```python
from build123d import *

# Parameters (mm, degrees)
F1_DEPTH    = 279.4
F2_T1_DEPTH = 136.906


# Not quite as in the source:
# - a fillet or chamfer that OpenCascade refuses, or shapes differently, is made with other operations: its cross-section is extruded or revolved along the edge and cut away or added


with BuildPart() as f1:
    # F0 (on Top) → F1 (new body)
    with BuildSketch(Plane.XY):
        with BuildLine():
            Line((49.403, -12.7), (49.403, 25.4))
            Line((49.403, 25.4), (10.7822931626, 25.4))
            Line((10.7822931626, 25.4), (25.44699, 0))
            Line((25.44699, 0), (-25.35301, 0))
            Line((-25.35301, 0), (-10.6883131626, 25.4))
            Line((-10.6883131626, 25.4), (-49.403, 25.4))
            Line((-49.403, 25.4), (-49.403, -12.7))
            ThreePointArc((-49.403, -12.7), (-45.6832561211, -21.6802561211), (-36.703, -25.4))
            Line((-36.703, -25.4), (36.703, -25.4))
            ThreePointArc((36.703, -25.4), (45.6832561211, -21.6802561211), (49.403, -12.7))
        make_face()
    extrude(amount=F1_DEPTH)

    # F2: fillet of radius 12.7 on 1 edges, made by hand

    # F2_s2 → F2_t1 (cut)
    with BuildSketch(Plane.YZ.offset(-68.453)):
        with BuildLine():
            ThreePointArc((-25.4, 266.7), (-21.6802561211, 275.6802561211), (-12.7, 279.4))
            Line((-12.7, 279.4), (-25.4, 279.4))
            Line((-25.4, 279.4), (-25.4, 266.7))
        make_face()
    extrude(amount=F2_T1_DEPTH, mode=Mode.SUBTRACT)


solid = f1.part
```
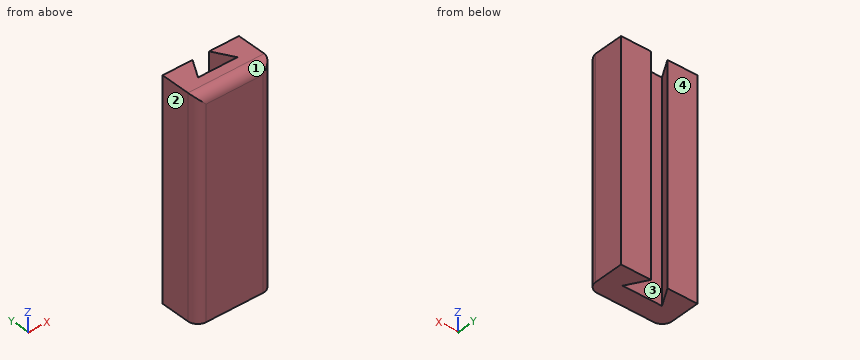
Check sheet for the modelled part. Datum: model origin and axes. Units: mm. Face numbers are marked on the shaded views. Round coordinates to 2 decimals unless told otherwise and drop trailing zeros. Order: outer loops, then holes, each group sorted by start corner. A loop starts at its lowest first (then second) coordinate and runs counter-clockwise, first axis right, second up. Notation, with made-up numbers: (58, 9) -> (68, 9) arc R25 ccw to (68, 27) -> close; hole circle Ø5 at (22.5, 8). An arc over 180 degrees is marked (long way). Use CSV: the item, a comma, the result in double quotes.
(1) Cross-section at A-A (y = 9). Record the boundary of the cut face in (x, z), and give its area (3 significant figures).
Worked out:
outline,"(-49.4, 0) -> (-20.16, 0) -> (-20.16, 279.4) -> (-49.4, 279.4) -> close; (20.25, 0) -> (49.4, 0) -> (49.4, 279.4) -> (20.25, 279.4) -> close"
area,"16,300 mm²"
(2) Draft check along Y on the marked faces 1, 2, 3 and 4. Enter one of: pulls with the +Y half, pulls with the -Y half, needs draft (parallel to the pull), parting line crosses it, or undercut.
Worked out:
face 1,"pulls with the -Y half"
face 2,"needs draft"
face 3,"undercut"
face 4,"pulls with the +Y half"
(3) Depth check by flat-ended pin: pin 1 (6 mm diameter, centred on x = 6.5, z = 82.5, fed in from +Y); pin 2 (2 mm diameter, centred on x = 16.5, y = -19.5, fed in from +Z); pin 3 (5 mm diameter, centred on y = -18, z = 75, fed in from -X). Enter the tip coordinate at first touch or a pass-through.
Worked out:
pin 1,"y = 0"
pin 2,"z = 278"
pin 3,"x = -49.09"
(4) Material ranges on line 1 along X through (y, z) = (19, 218.5); line 2 along Y through (x, z) = (0.5, 182); line 3 along Z through (x, y) = (-42, -13.5), recorded low to high. Write a range as from..to.
Worked out:
line 1,"-49.4..-14.38, 14.48..49.4"
line 2,"-25.4..0"
line 3,"0..279.37"
(5) Cross-section at D-D (x = 20). Record the boundary of the cut face in (y, z), and give its area (3 significant figures).
Worked out:
outline,"(-25.4, 0) -> (0, 0) -> (0, 279.4) -> (-12.7, 279.4) arc R12.7 ccw to (-25.4, 266.7) -> close; (9.43, 0) -> (25.4, 0) -> (25.4, 279.4) -> (9.43, 279.4) -> close"
area,"11,500 mm²"
(6) Cross-section at C-C (x = -15.5). Record the boundary of the cut face in (y, z).
Worked out:
outline,"(-25.4, 0) -> (0, 0) -> (0, 279.4) -> (-12.7, 279.4) arc R12.7 ccw to (-25.4, 266.7) -> close; (17.07, 0) -> (25.4, 0) -> (25.4, 279.4) -> (17.07, 279.4) -> close"
(7) Cross-section at B-B (z = 137). Record the boundary of the cut face in (x, y), and give its area (3 significant figures).
Worked out:
outline,"(-49.4, -12.7) arc R12.7 ccw to (-36.7, -25.4) -> (36.7, -25.4) arc R12.7 ccw to (49.4, -12.7) -> (49.4, 25.4) -> (10.78, 25.4) -> (25.45, 0) -> (-25.35, 0) -> (-10.69, 25.4) -> (-49.4, 25.4) -> close"
area,"4,030 mm²"
